Answer from the drawing. Dimensions are ordinates in mm from the lowest x, y and z of the part. Give positions to 0.01 mm unless a question says otherwise; leave off trailing zeros. Loops run counter-clockwise (first coordinate to the right, second up) from the corner with the lowest first, then second, coordinate; pieces in that order, holes last. Notation, with made-up numbers: (27, -16.5) -> (49, -16.5) arc R18 ccw to (49, 17.5) -> close; hole circle Ø2 at (73.25, 50.5). An arc over 180 degrees is marked (long way). Write each question's results on one line, items separated by ' | '. Start each with the question number.
Item 1: This flat-tipped pin is pushed along its axis until it touches: P1, Ø4, axis at x = 88.9, y = 12.7, coming from the +Z side. Where does it stop, or does it pass through?
Item 2: Section B-B on x = 12.7 is taken. Write down the section's boundary in (y, z) (1 decimal).
Item 3: Section A-A on x = 63.5 is taken. Write down the section's boundary in (y, z) (1 decimal).
Item 4: Section D-D on z = 3.85 is taken. Write down the section's boundary in (x, y).
Item 5: Find the intervals of material crossed by line 1 (Y direction, x = 12.7, z = 3.15); line 2 (Y direction, x = 10, z = 2) (1 decimal); line 3 (X direction, y = 11, z = 1), in increasing order.
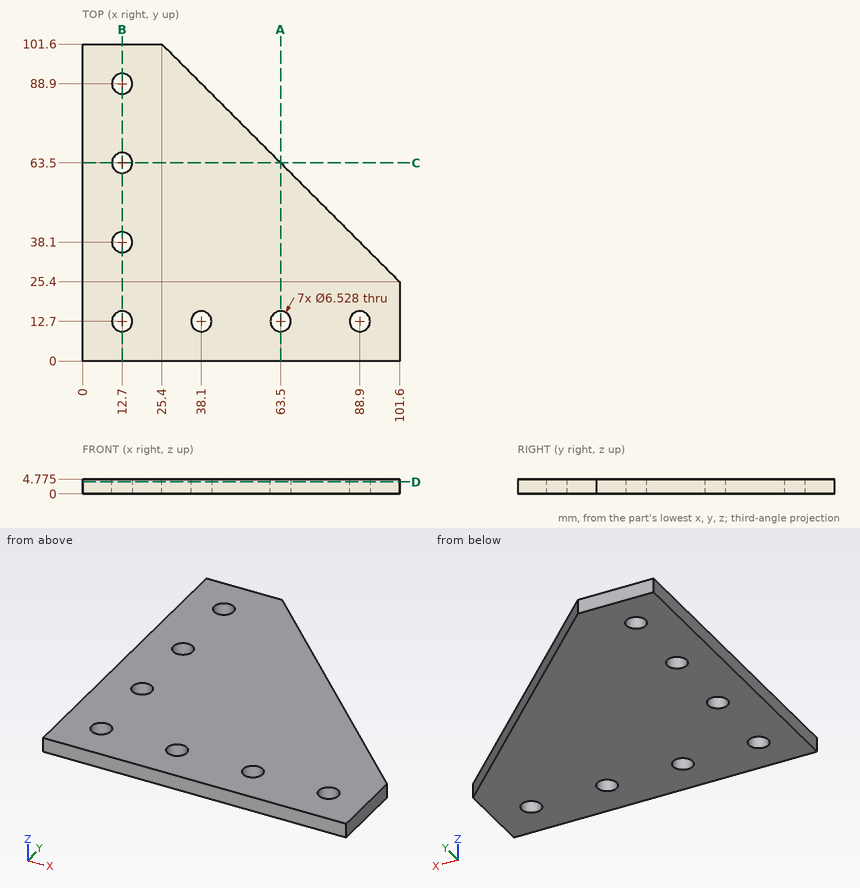
Findings:
1) P1: through
2) outline: (0, 0) -> (9.4, 0) -> (9.4, 4.8) -> (0, 4.8) -> close; (16, 0) -> (34.8, 0) -> (34.8, 4.8) -> (16, 4.8) -> close; (41.4, 0) -> (60.2, 0) -> (60.2, 4.8) -> (41.4, 4.8) -> close; (66.8, 0) -> (85.6, 0) -> (85.6, 4.8) -> (66.8, 4.8) -> close; (92.2, 0) -> (101.6, 0) -> (101.6, 4.8) -> (92.2, 4.8) -> close
3) outline: (0, 0) -> (9.4, 0) -> (9.4, 4.8) -> (0, 4.8) -> close; (16, 0) -> (63.5, 0) -> (63.5, 4.8) -> (16, 4.8) -> close
4) outline: (0, 0) -> (101.6, 0) -> (101.6, 25.4) -> (25.4, 101.6) -> (0, 101.6) -> close; hole circle Ø6.53 at (12.7, 12.7); hole circle Ø6.53 at (12.7, 38.1); hole circle Ø6.53 at (12.7, 63.5); hole circle Ø6.53 at (12.7, 88.9); hole circle Ø6.53 at (38.1, 12.7); hole circle Ø6.53 at (63.5, 12.7); hole circle Ø6.53 at (88.9, 12.7)
5) line 1: 0 to 9.44, 15.96 to 34.84, 41.36 to 60.24, 66.76 to 85.64, 92.16 to 101.6 | line 2: 0 to 10.9, 14.5 to 36.3, 39.9 to 61.7, 65.3 to 87.1, 90.7 to 101.6 | line 3: 0 to 9.91, 15.49 to 35.31, 40.89 to 60.71, 66.29 to 86.11, 91.69 to 101.6
